```python
from build123d import *

# Parameters (mm, degrees)
SKETCH1_W           = 43
SKETCH1_H           = 20
BOSS_EXTRUDE1_DEPTH = 1.6
SKETCH2_R           = 8
BOSS_EXTRUDE2_DEPTH = 13


with BuildPart() as part:
    # Sketch1 → Boss-Extrude1 (new body)
    with BuildSketch(Plane.XY):
        Rectangle(SKETCH1_W, SKETCH1_H)
    extrude(amount=BOSS_EXTRUDE1_DEPTH)

    # Sketch2 → Boss-Extrude2 (add)
    with BuildSketch(Plane.XY.offset(1.6)):
        with Locations(Location((-11.5, 0, 0), (0, 0, 180))):
            Circle(SKETCH2_R)
        with Locations(Location((11.5, 0, 0), (0, 0, 180))):
            Circle(SKETCH2_R)
    extrude(amount=BOSS_EXTRUDE2_DEPTH)


solid = part.part
```
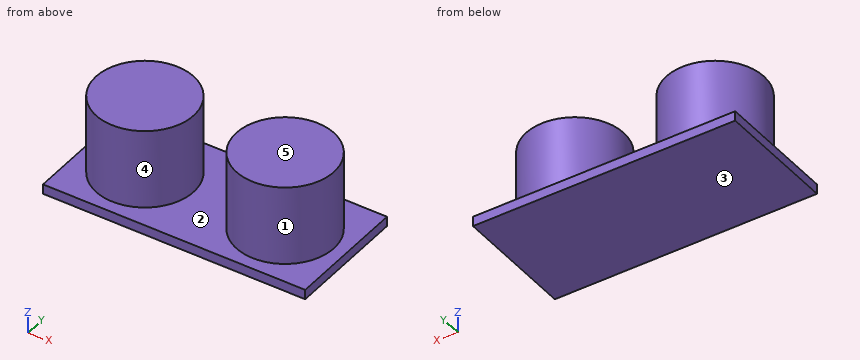
Work out the finished part from the listing and answer in its coordinate system (mm). Face numbers are marked on the shaded views. A direction names the side the tool comes from. Coordinates: 2 decimals unless noted, no trailing zeros. Write each loop counter-clockwise with the first axis right and the second up, starting at its lowest first coordinate (ties: lowest second). Pieces come first, ordered by that corner, then holes.
Q1. Each of these flat-tipped pins is pushed along its axis until it touches: pin 1 Ø6 at (y, z) = (-7, 13) entering from +X; pin 2 Ø6 at (x, y) = (-4, 4) entering from +Z; pin 3 Ø1.5 at (y, z) = (-4.5, 2.5) entering from +X; pin 4 Ø5 at (x, z) = (9, 11.5) entering from -Y. Where does it stop, or does it pass through?
Q2. Which of the six approach directions +Z, -Z, +X, -X, +Y, -Y give full straight-line access (tool end or side, diameter ignored) to the marked faces 4 and 5?
Q3. A cutting plane is placed at D-D, the plane x = -8.5. Give the vertices of the cut face in (y, z).
Q4. A cutting plane is placed at B-B, the plane y = 0. Give the vertices of the cut face in (x, z), then the cut area to 3 significant figures.
Q5. Find the intervals of material crossed by line 1 (X direction, y = 0.25, z = 5.5); line 2 (Z direction, x = -1.5, y = 1.25); line 3 (X direction, y = 1, z = 6.5), in increasing order.
Q6. Determine the mould class of the marked faces 1, 2 and 3 for opening direction X: released by +X, released by -X, zero draft, split by the parting line, or undercut.
Q7. A cutting plane is placed at A-A, the plane x = 11.5. Give the vertices of the cut face in (y, z).
Q8. A cutting plane is placed at C-C, the plane z = 9.5. Give the vertices of the cut face in (x, y).
Findings below:
1. pin 1: stops at x = 18.43
1. pin 2: stops at z = 14.6
1. pin 3: stops at x = 18.57
1. pin 4: stops at y = -8
2. face 4: +Z
2. face 5: +Z, +X, -X, +Y, -Y
3. outline: (-10, 0) - (10, 0) - (10, 1.6) - (7.42, 1.6) - (7.42, 14.6) - (-7.42, 14.6) - (-7.42, 1.6) - (-10, 1.6) - close
4. outline: (-21.5, 0) - (21.5, 0) - (21.5, 1.6) - (19.5, 1.6) - (19.5, 14.6) - (3.5, 14.6) - (3.5, 1.6) - (-3.5, 1.6) - (-3.5, 14.6) - (-19.5, 14.6) - (-19.5, 1.6) - (-21.5, 1.6) - close
4. area: 485 mm2
5. line 1: x = -19.5 to -3.5, 3.5 to 19.5
5. line 2: z = 0 to 1.6
5. line 3: x = -19.44 to -3.56, 3.56 to 19.44
6. face 1: undercut
6. face 2: undercut
6. face 3: zero draft
7. outline: (-10, 0) - (10, 0) - (10, 1.6) - (8, 1.6) - (8, 14.6) - (-8, 14.6) - (-8, 1.6) - (-10, 1.6) - close
8. outline: circle Ø16 at (-11.5, 0); circle Ø16 at (11.5, 0)
